Geometry check sheet. Reference: the model listing, model coordinates, mm. A direction names the side the tool comes from. Round coordinates to 2 decimals unless told otherwise and drop trailing zeros. Order: outer loops, then holes, each group sorted by start corner. A loop starts at its lowest first (then second) coordinate and runs counter-clockwise, first axis right, second up.
(1) Gauge pin test, flat ends, axial feed: P1, Ø4, axis at y = -82.5, z = -82.5, coming from the -X side; P2, Ø2, axis at x = 688, y = -73.5, coming from the +Z side; P3, Ø3, axis at y = 4, z = -221, coming from the +X side. Record the tip position at first contact, or that the pin passes through.
(2) Set-up check for faces 1 (the face through (373, -31, -31.75)), 2 (the face through (363.1, 22.7, 22.2)): record each of +Z, -Z, +X, -X, +Y, -Y from which the full face is reachable in a straight line by a thin tool's end or side.
(3) Draft check along X on faces 3 (the face through (0, -31, -212)), 4 (the face through (363, -31, 31.75)), 5 (the face through (-53.95, -86.2, -211.76)). Enter one of: pulls with the +X half, pulls with the -X half, needs draft (parallel to the pull), parting line crosses it, or undercut.
(4) Cross-section at A-A on z = -280. Enter the section's corners in (x, y), and give its area (3 significant figures).
(5) Thickness scan on L1, parallel to X at y = -14, z = -138.5; L2, parallel to Z at x = 628.5, y = -10. Record the ranges inside material, lowest first.
(6) Cross-section at D-D on y = 18. Enter the section's corners in (x, z) (3 decimals).
(7) Cross-section at C-C on x = 681. Enter the section's corners in (y, z).
(8) Cross-section at B-B on y = -31.5. Enter the section's corners in (x, z) (3 decimals), and give its area (3 significant figures).
from build123d import *

# Parameters (mm, degrees)
BOSS_EXTRUDE1_DEPTH = 736.6
REVOLVE13_ANGLE     = 90
REVOLVE12_ANGLE     = 90
BOSS_EXTRUDE3_DEPTH = 736.6
REVOLVE2_ANGLE      = 90
SKETCH9_R           = 31.75
BOSS_EXTRUDE4_DEPTH = 736.6
REVOLVE10_ANGLE     = 90
BOSS_EXTRUDE5_DEPTH = 736.6
SKETCH16_W          = 434.975
SKETCH16_H          = 127
CUT_EXTRUDE1_DEPTH  = 1203.851588934


with BuildPart() as part:
    # Sketch1 → Boss-Extrude1 (new body)
    with BuildSketch(Plane(origin=(0, 0, 0), x_dir=(0, 0, -1), z_dir=(1, 0, 0))):
        with BuildLine():
            Line((-31.75, 0), (-31.75, -63.5))
            ThreePointArc((-31.75, -63.5), (-22.450640303, -85.950640303), (0, -95.25))
            Line((0, -95.25), (31.75, -95.25))
            Line((31.75, -95.25), (31.75, 0))
            Line((31.75, 0), (31.75, 31.75))
            Line((31.75, 31.75), (0, 31.75))
            ThreePointArc((0, 31.75), (-22.450640303, 22.450640303), (-31.75, 0))
        make_face()
    extrude(amount=BOSS_EXTRUDE1_DEPTH)



with BuildPart() as body_2:
    # Sketch8 → Revolve13 (revolve)
    with BuildSketch(Plane(origin=(736.6, 0, 0), x_dir=(0, 0, -1), z_dir=(1, 0, 0))):
        with BuildLine():
            Line((-31.75, 0), (-31.75, -63.5))
            ThreePointArc((-31.75, -63.5), (-22.450640303, -85.950640303), (0, -95.25))
            Line((0, -95.25), (31.75, -95.25))
            Line((31.75, -95.25), (31.75, 31.75))
            Line((31.75, 31.75), (0, 31.75))
            ThreePointArc((0, 31.75), (-22.450640303, 22.450640303), (-31.75, 0))
        make_face()
    revolve(axis=Axis((736.6, -95.25, -31.75), (0, 1, 0)), revolution_arc=REVOLVE13_ANGLE)


with BuildPart() as body_3:
    # Sketch15 → Revolve12 (revolve)
    with BuildSketch(Plane(origin=(0, 0, -31.75), x_dir=(0, 0, 1), z_dir=(-1, 0, 0))):
        with BuildLine():
            Line((63.5, -63.5), (63.5, 0))
            ThreePointArc((63.5, 0), (54.200640303, 22.450640303), (31.75, 31.75))
            Line((31.75, 31.75), (0, 31.75))
            Line((0, 31.75), (0, -95.25))
            Line((0, -95.25), (31.75, -95.25))
            ThreePointArc((31.75, -95.25), (54.200640303, -85.950640303), (63.5, -63.5))
        make_face()
    revolve(axis=Axis((0, 31.75, -31.75), (0, -1, 0)), revolution_arc=REVOLVE12_ANGLE)


with BuildPart() as part_1:
    add(part.part)

    add(body_2.part)  # Boss-Extrude3 merges body 2
    # Sketch7 → Boss-Extrude3 (add)
    with BuildSketch(Plane(origin=(0, 0, -31.75), x_dir=(-1, 0, 0), z_dir=(0, 0, -1))):
        with BuildLine():
            Line((-800.1, 0), (-800.1, -63.5))
            ThreePointArc((-800.1, -63.5), (-790.800640303, -85.950640303), (-768.35, -95.25))
            Line((-768.35, -95.25), (-736.6, -95.25))
            Line((-736.6, -95.25), (-736.6, 31.75))
            Line((-736.6, 31.75), (-768.35, 31.75))
            ThreePointArc((-768.35, 31.75), (-790.800640303, 22.450640303), (-800.1, 0))
        make_face()
    extrude(amount=BOSS_EXTRUDE3_DEPTH)

    # Sketch12 → Revolve2 (revolve)
    with BuildSketch(Plane(origin=(1454.15, 0, -768.35), x_dir=(-1, 0, 0), z_dir=(0, 0, -1))):
        with BuildLine():
            Line((654.05, 0), (654.05, -63.5))
            ThreePointArc((654.05, -63.5), (663.349359697, -85.950640303), (685.8, -95.25))
            Line((685.8, -95.25), (717.55, -95.25))
            Line((717.55, -95.25), (717.55, 31.75))
            Line((717.55, 31.75), (685.8, 31.75))
            ThreePointArc((685.8, 31.75), (663.349359697, 22.450640303), (654.05, 0))
        make_face()
    revolve(axis=Axis((736.6, -95.25, -768.35), (0, 1, 0)), revolution_arc=REVOLVE2_ANGLE)


    add(body_3.part)  # Boss-Extrude4 merges body 3
    # Sketch9 → Boss-Extrude4 (add)
    with BuildSketch(Plane(origin=(0, 0, -31.75), x_dir=(-1, 0, 0), z_dir=(0, 0, -1))):
        with BuildLine():
            ThreePointArc((0, 4.4e-08), (9.299359713, 22.450640318), (31.75, 31.75))
            Line((31.75, 31.75), (0, 31.75))
            Line((0, 31.75), (0, 4.4e-08))
        make_face()
        with Locations((31.75, 0)):
            Circle(SKETCH9_R)
        with BuildLine():
            ThreePointArc((31.75, -31.75), (9.299359682, -22.450640287), (0, 4.4e-08))
            Line((0, 4.4e-08), (0, -63.500000004))
            ThreePointArc((0, -63.500000004), (9.299359696, -41.049359699), (31.75, -31.75))
        make_face()
        with BuildLine():
            Line((63.5, -63.5), (63.5, 0))
            ThreePointArc((63.5, 0), (54.200640303, -22.450640303), (31.75, -31.75))
            ThreePointArc((31.75, -31.75), (54.200640303, -41.049359697), (63.5, -63.5))
        make_face()
        with Locations((31.75, -63.5)):
            Circle(SKETCH9_R)
        with BuildLine():
            ThreePointArc((31.75, -95.25), (9.299359699, -85.950640304), (0, -63.500000004))
            Line((0, -63.500000004), (0, -95.25))
            Line((0, -95.25), (31.75, -95.25))
        make_face()
    extrude(amount=BOSS_EXTRUDE4_DEPTH)


with BuildPart() as body_2_2:
    # Sketch14 → Revolve10 (revolve)
    with BuildSketch(Plane(origin=(0, 0, -768.35), x_dir=(-1, 0, 0), z_dir=(0, 0, -1))):
        with BuildLine():
            Line((31.75, 31.75), (0, 31.75))
            Line((0, 31.75), (0, -95.25))
            Line((0, -95.25), (31.75, -95.25))
            ThreePointArc((31.75, -95.25), (54.200640303, -85.950640303), (63.5, -63.5))
            Line((63.5, -63.5), (63.5, 0))
            ThreePointArc((63.5, 0), (54.200640303, 22.450640303), (31.75, 31.75))
        make_face()
    revolve(axis=Axis((0, 31.75, -768.35), (0, -1, 0)), revolution_arc=REVOLVE10_ANGLE)


with BuildPart() as body_3_2:
    # Sketch10 → Boss-Extrude5 (new body)
    with BuildSketch(Plane(origin=(0, 0, 0), x_dir=(0, 0, -1), z_dir=(1, 0, 0))):
        with BuildLine():
            Line((800.1, 31.75), (768.35, 31.75))
            Line((768.35, 31.75), (768.35, -95.25))
            Line((768.35, -95.25), (800.1, -95.25))
            ThreePointArc((800.1, -95.25), (822.550640303, -85.950640303), (831.85, -63.5))
            Line((831.85, -63.5), (831.85, 0))
            ThreePointArc((831.85, 0), (822.550640303, 22.450640303), (800.1, 31.75))
        make_face()
    extrude(amount=BOSS_EXTRUDE5_DEPTH)


with BuildPart() as part_2:
    add(part_1.part)

    # Combine1: union body 3 2, body 2 2
    add(body_3_2.part)
    add(body_2_2.part)

    # Sketch16 → Cut-Extrude1 (cut, through all)
    with BuildSketch(Plane(origin=(800.1, 0, 0), x_dir=(0, 0, -1), z_dir=(1, 0, 0))):
        with Locations((614.3625, -31.75)):
            Rectangle(SKETCH16_W, SKETCH16_H)
    extrude(amount=-CUT_EXTRUDE1_DEPTH, mode=Mode.SUBTRACT)


solid = part_2.part
Found:
1. P1: stops at x = -58.57
1. P2: stops at z = 30.45
1. P3: stops at x = 800
2. face 1: -Z, +Y, -Y
2. face 2: +Z, +X, -X, +Y
3. face 3: undercut
3. face 4: needs draft
3. face 5: pulls with the -X half
4. outline: (-63.5, -63.5) arc R31.75 ccw to (-31.75, -95.25) - (0, -95.25) - (0, 31.75) - (-31.75, 31.75) arc R31.75 ccw to (-63.5, 0) - close; (736.6, -95.25) - (768.35, -95.25) arc R31.75 ccw to (800.1, -63.5) - (800.1, 0) arc R31.75 ccw to (768.35, 31.75) - (736.6, 31.75) - close
4. area: 15,300 mm2
5. L1: x = -63.5 to 0, 736.6 to 800.1
5. L2: z = -31.75 to 31.75
6. outline: (-57.905, -396.875) - (0, -396.875) - (0, -31.75) - (736.6, -31.75) - (736.6, -396.875) - (794.505, -396.875) - (794.505, -31.75) arc R57.905 ccw to (736.6, 26.155) - (0, 26.155) arc R57.905 ccw to (-57.905, -31.75) - close
7. outline: (-95.25, -31.75) - (31.75, -31.75) - (31.75, 0) arc R31.75 ccw to (0, 31.75) - (-63.5, 31.75) arc R31.75 ccw to (-95.25, 0) - close
8. outline: (-63.5, -396.875) - (0, -396.875) - (0, -31.75) - (736.6, -31.75) - (736.6, -396.875) - (800.1, -396.875) - (800.1, -31.75) arc R63.5 ccw to (736.6, 31.75) - (0, 31.75) arc R63.5 ccw to (-63.5, -31.75) - close
8. area: 99,500 mm2
